Check sheet for the drawn part. Datum: minimum x, y, z corner. Units: mm. Coordinates: 2 decimals unless noted, no trailing zeros. Write each loop counter-clockwise with the first axis right and the second up, starting at its lowest first coordinate (ties: lowest second). Pieces come first, ordered by that corner, then holes. Notation, with made-up numbers: (75, 10.5) -> (116, 10.5) arc R13 cw to (116, 15.5) -> close; hole circle Ø6 at (60, 30). An arc over 180 degrees is marked (long way). Answer in a Markdown table with one row per item. Add a question column.
1. Depth check by flat-ended pin: P1, Ø4, axis at y = 17.5, z = 4.5, coming from the -X side. Enter the tip coordinate at first touch or a pass-through.
2. Scan lines: L1, parallel to Y at x = 56, z = 23 (1 decimal); L2, parallel to X at y = 67, z = 12 (1 decimal); L3, parallel to Y at x = 37, z = 4 (1 decimal). Record each from-to range of solid material in increasing order. Write a range as from..to.
3. Cross-section at D-D on x = 99. Record the cut outline in (y, z), and give its area (3 significant figures).
4. Cross-section at A-A on x = 61. Record the cut outline in (y, z) (1 decimal), and give its area (3 significant figures).
5. Cross-section at B-B on y = 27. Record the cut outline in (x, z).
6. Mould release check, pull along Y, two halves, no side actions. Record for the marked faces 1, 2, 3 and 4: pulls with the +Y half, pulls with the -Y half, needs draft (parallel to the pull), parting line crosses it, or undercut.
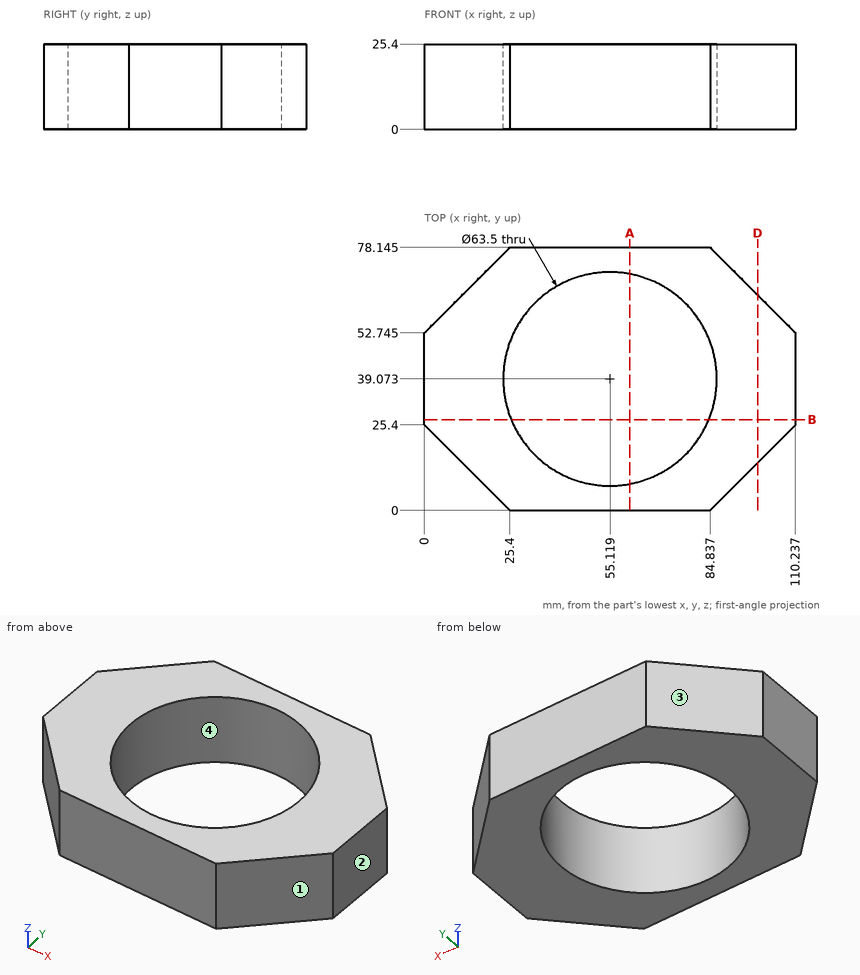
Results found:
| question | item | result |
|---|---|---|
| 1 | P1 | stops at x = 5.9 |
| 2 | L1 | y = 0..7.3, 70.8..78.1 |
| 2 | L2 | x = 14.3..40, 70.2..96 |
| 2 | L3 | y = 0..13, 65.1..78.1 |
| 3 | outline | (14.16, 0) -> (63.98, 0) -> (63.98, 25.4) -> (14.16, 25.4) -> close |
| 3 | area | 1,270 mm^2 |
| 4 | outline | (0, 0) -> (7.9, 0) -> (7.9, 25.4) -> (0, 25.4) -> close; (70.3, 0) -> (78.1, 0) -> (78.1, 25.4) -> (70.3, 25.4) -> close |
| 4 | area | 400 mm^2 |
| 5 | outline | (0, 0) -> (25.75, 0) -> (25.75, 25.4) -> (0, 25.4) -> close; (84.48, 0) -> (110.24, 0) -> (110.24, 25.4) -> (84.48, 25.4) -> close |
| 6 | face 1 | pulls with the -Y half |
| 6 | face 2 | needs draft |
| 6 | face 3 | pulls with the +Y half |
| 6 | face 4 | undercut |
